```python
from build123d import *

# Parameters (mm, degrees)
F0_R     = 4.9
F0_R_2   = 17.5
F0_R_3   = 11.15
F1_DEPTH = 7
F2_R     = 2


with BuildPart() as f1:
    # F0 (on Top) → F1 (new body)
    with BuildSketch(Plane.XY):
        Polygon((22.643075, 17.802371), (4.095768, 28.510664), (4.234027, 40.684762), (-9.416056, 40.839784), (-9.263652, 54.259394), (-31.028777, 53.743419), (-42.358188, 35.152255), (-30.660262, 28.574436), (-37.351051, 16.675606), (-26.738843, 10.708293), (-26.738843, -10.708293), (-37.351051, -16.675606), (-30.660262, -28.574436), (-42.358188, -35.152255), (-31.028777, -53.743419), (-9.263652, -54.259394), (-9.416056, -40.839784), (4.234027, -40.684762), (4.095768, -28.510664), (22.643075, -17.802371), (33.117024, -24.009156), (40.076318, -12.265348), (51.62184, -19.107139), (61.241437, 0), (51.62184, 19.107139), (40.076318, 12.265348), (33.117024, 24.009156), align=None)
        with Locations((-21.059453, -36.476043)):
            Circle(F0_R, mode=Mode.SUBTRACT)
        Circle(F0_R_2, mode=Mode.SUBTRACT)
        with Locations((42.118907, 0)):
            Circle(F0_R, mode=Mode.SUBTRACT)
        with Locations((-21.059453, 36.476043)):
            Circle(F0_R, mode=Mode.SUBTRACT)
        Circle(F0_R_2)
        Circle(F0_R_3, mode=Mode.SUBTRACT)
    extrude(amount=F1_DEPTH)

    # F2
    f2_edges = [f1.edges().sort_by_distance(p)[0] for p in [
        (13.369421, -23.156517, 7),
        (27.88005, -20.905763, 7),
        (36.596671, -18.137252, 7),
        (45.849079, -15.686243, 7),
        (56.431638, -9.553569, 7),
        (56.431638, 9.553569, 7),
        (45.849079, 15.686243, 7),
        (36.596671, 18.137252, 7),
        (27.88005, 20.905763, 7),
        (13.369421, 23.156517, 7),
        (4.164897, 34.597713, 7),
        (-2.591015, 40.762273, 7),
        (-9.339854, 47.549589, 7),
        (-36.693482, 44.447837, 7),
        (-20.146215, 54.001407, 7),
        (-36.509225, 31.863346, 7),
        (-34.005657, 22.625021, 7),
        (-32.044947, 13.69195, 7),
        (-26.738843, 0, 7),
        (-32.044947, -13.69195, 7),
        (-34.005657, -22.625021, 7),
        (-36.509225, -31.863346, 7),
        (-36.693482, -44.447837, 7),
        (-20.146215, -54.001407, 7),
        (-2.591015, -40.762273, 7),
        (4.164897, -34.597713, 7),
        (-9.339854, -47.549589, 7),
        (-20.146215, -54.001407, 0),
        (-36.693482, -44.447837, 0),
        (-9.339854, -47.549589, 0),
        (-2.591015, -40.762273, 0),
        (4.164897, -34.597713, 0),
        (13.369421, -23.156517, 0),
        (27.88005, -20.905763, 0),
        (36.596671, -18.137252, 0),
        (45.849079, -15.686243, 0),
        (56.431638, -9.553569, 0),
        (56.431638, 9.553569, 0),
        (45.849079, 15.686243, 0),
        (36.596671, 18.137252, 0),
        (13.369421, 23.156517, 0),
        (4.164897, 34.597713, 0),
        (-9.339854, 47.549589, 0),
        (-2.591015, 40.762273, 0),
        (-20.146215, 54.001407, 0),
        (-36.509225, -31.863346, 0),
        (-34.005657, -22.625021, 0),
        (-32.044947, -13.69195, 0),
        (-26.738843, 0, 0),
        (-32.044947, 13.69195, 0),
        (-34.005657, 22.625021, 0),
        (-36.509225, 31.863346, 0),
        (-36.693482, 44.447837, 0),
    ]]
    fillet(f2_edges, radius=F2_R)


solid = f1.part
```
Check sheet for the modelled part. Datum: model origin and axes. Units: mm. A direction names the side the tool comes from. Give positions to 0.01 mm unless a question says otherwise; leave off trailing zeros. Use CSV: the item, a comma, the result in double quotes. Start each with the question number.
1) Sectioned sample at A-A, the plane z = 3.5. Give the number of separate pieces and of enclosed holes in the cut face, plus the area to 3 significant figures.
2) Set-up check for faces 1 (the face through (-19.98, -53.435, 6.399)), 2 (the face through (27.748, -20.165, 0.601)), 3 (the face through (36.548, -18.219, 3.479)), 4 (the face through (36.67, -16.89, 6.4)), 5 (the face through (27.59, 20.07, 6.4)): record each of +Z, -Z, +X, -X, +Y, -Y from which the full face is reachable in a straight line by a thin tool's end or side.
3) Material ranges on line 1 (Y direction, x = -35.5, z = 5.5); line 2 (X direction, y = -4.5, z = 2.5); line 3 (X direction, y = 15, z = 0.5), recorded low to high. Write a range as from..to.
4) Mould release check, pull along X, two halves, no side actions. Record for faces 6 (the face through (45.37, -14.74, 6.4)), 7 (the face through (-13, 1, 0)), 8 (the face through (-32.965, -23.313, 6.399)): released by +X, released by -X, zero draft, split by the parting line, or undercut.
5) Go/stop test with flat-tipped pins: P1, Ø1.5, axis at y = 4.5, z = 4, coming from the -X side; P2, Ø1, axis at x = 45, z = 3, coming from the -Y side; P3, Ø15.5, axis at x = 42.12, y = 0, coming from the -Z side; P4, Ø2, axis at y = -26.5, z = 1, coming from the -X side. Record where each tip stops, or that it passes through.
Recorded:
1,separate pieces,"1"
1,enclosed holes,"4"
1,area,"5,190 mm2"
2,face 1,"+Z, -X, -Y"
2,face 2,"-Z, -Y"
2,face 3,"+Z, -Z, -Y"
2,face 4,"+Z, -Y"
2,face 5,"+Z, +Y"
3,line 1,"-46.28..-31.37, -19.84..-15.71, 15.71..19.84, 31.37..46.28"
3,line 2,"-26.74..-10.2, 10.2..40.18, 44.06..58.98"
3,line 3,"-32.99..37.67, 46.02..52.93"
4,face 6,"undercut"
4,face 7,"zero draft"
4,face 8,"released by -X"
5,P1,"x = -26.74"
5,P2,"y = -15.48"
5,P3,"z = 0"
5,P4,"x = -32.24"
